Geometry check sheet. Reference: the model listing, model coordinates, mm. Face numbers are marked on the shaded views. A direction names the side the tool comes from. Round coordinates to 2 decimals unless told otherwise and drop trailing zeros. Loops run counter-clockwise (first coordinate to the right, second up) from the corner with the lowest first, then second, coordinate; pieces in that order, holes last. Notation, with made-up numbers: (86, 43.25) -> (99, 43.25) arc R15 ccw to (99, 61.25) -> close; hole circle Ø3 at (8.5, 18). An arc over 180 degrees is marked (long way). Use a Markdown table: item, result. Add a question column.
Q1. Sectioned sample at A-A, the plane y = 12.7. Enter the section's corners in (x, z) (3 decimals), then the cut area to 3 significant figures.
Q2. Sectioned sample at B-B, the plane x = 6.35. Enter the section's corners in (y, z) (3 decimals), then the cut area to 3 significant figures.
Q3. Set-up check for the marked faces 1, 2 and 3: record each of +Z, -Z, +X, -X, +Y, -Y from which the full face is reachable in a straight line by a thin tool's end or side.
Q4. Gauge pin test, flat ends, axial feed: P1, Ø3, axis at x = 6.35, z = -88.9, coming from the -Y side; P2, Ø12.5, axis at x = 16.5, y = 43, coming from the -Z side; P3, Ø8, axis at x = 12.5, z = -26, coming from the -Y side; P4, Ø10, axis at x = 4, z = -52, coming from the -Y side (3 decimals). Record the tip position at first contact, or that the pin passes through.
Q5. Sectioned sample at C-C, the plane z = -88.9. Enter the section's corners in (x, y) (3 decimals), then the cut area to 3 significant figures.
Q6. Material ranges on L1, parallel to X at y = 12.7, z = -1.8; L2, parallel to Y at x = 6.35, z = -2.5; L3, parallel to Z at x = 6.35, y = 100.7, recorded low to high.
Q7. Sectioned sample at D-D, the plane y = 93. Enter the section's corners in (x, z) (3 decimals), then the cut area to 3 significant figures.
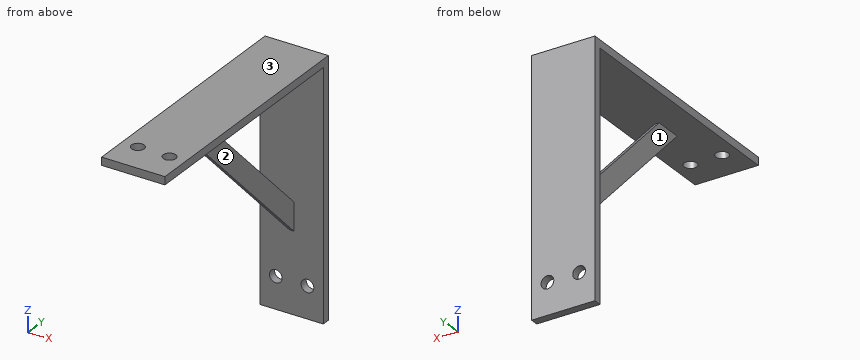
Autodesk Inventor part; units mm, degrees
ref_plane "Work Plane1" through (12.7, 0, 0) normal (1, 0, 0) x (0, 0, -1)
ref_plane "YZ Plane" through (0, 0, 0) normal (1, 0, 0) x (0, 1, 0)
ref_plane "XZ Plane" through (0, 0, 0) normal (0, 1, 0) x (-1, 0, 0)
sketch "Sketch1" plane through (0, 0, 0) normal (1, 0, 0) x (0, 1, 0)
  line L0 (0, 0) -> (101.6, 0)
  line L1 (101.6, 0) -> (101.6, -101.6)
  line L2 (98.425, -101.6) -> (98.425, -3.175)
  line L3 (98.425, -3.175) -> (0, -3.175)
  line L4 (101.6, -101.6) -> (98.425, -101.6)
  line L5 (0, 0) -> (0, -3.175)
  dimension "d0" = 101.6
  dimension "d1" = 101.6
  dimension "d2" = 3.175
extrude "Extrusion1" add sketch "Sketch1" along normal blind 25.4
ref_plane "Work Plane1" through (12.7, 0, 0) normal (1, 0, 0) x (0, 0, -1)
sketch "Sketch2" plane through (12.7, 0, 0) normal (1, 0, 0) x (0, 0, -1)
  line L0 (2.312, 31.3076) -> (70.5907, 99.5863)
  line L1 (2.312, 31.3076) -> (98.8727, 31.3076) construction
  line L2 (59.3736, 99.5863) -> (2.312, 42.5247)
  line L3 (70.5907, 99.5863) -> (59.3736, 99.5863)
  line L4 (2.312, 31.3076) -> (2.312, 42.5247)
  point P0 (0, 0)
  dimension "d6" = 45
  dimension "d7" = 7.9317
extrude "Extrusion2" add sketch "Sketch2" along normal mid plane 1.778
sketch "Sketch4" plane through (0, 98.425, -101.6) normal (0, -1, 0) x (1, 0, 0)
  line L0 (0, 0) -> (0, 98.425)
  line L1 (0, 0) -> (25.4, 0)
  circle A0 centre (6.35, 12.7) radius 2.2746
  circle A1 centre (19.05, 12.7) radius 2.2746
  point P0 (0, 101.6)
  dimension "d10" = 12.7
  dimension "d11" = 6.35
  dimension "d14" = 12.7
hole "Hole1" at (19.05, 98.425, -88.9) at (6.35, 98.425, -88.9) direction (0, 1, 0) diameter 5.1054 depth 25.4 tip angle 118
sketch "Sketch5" plane through (0, 0, -3.175) normal (0, 0, -1) x (-1, 0, 0)
  line L0 (-25.4, 0) -> (-25.4, 98.425)
  line L1 (0, 0) -> (-25.4, 0)
  circle A0 centre (-19.05, 12.7) radius 2.2861
  circle A1 centre (-6.35, 12.7) radius 2.2861
  dimension "d26" = 12.7
  dimension "d27" = 6.35
  dimension "d30" = 12.7
hole "Hole2" at (19.05, 12.7, -3.175) at (6.35, 12.7, -3.175) direction (0, 0, 1) diameter 5.1054 depth 25.4 tip angle 118
equation "\"d11\" = 0.25 * d3"
equation "\"d14\" = 0.5 * d3"
equation "\"d27\" = 0.25 * d3"
equation "\"d30\" = 0.5 * d3"
equation "\"d5\" = -0.5 * d3"
properties part number "angleBracket"
Values:
| question | item | result |
|---|---|---|
| 1 | outline | (0, -3.175) -> (3.797, -3.175) -> (3.797, 0) -> (0, 0) -> close; (8.903, -3.175) -> (16.497, -3.175) -> (16.497, 0) -> (8.903, 0) -> close; (21.603, -3.175) -> (25.4, -3.175) -> (25.4, 0) -> (21.603, 0) -> close |
| 1 | area | 48.2 mm^2 |
| 2 | outline | (0, -3.175) -> (10.147, -3.175) -> (10.147, 0) -> (0, 0) -> close; (15.253, -3.175) -> (98.425, -3.175) -> (98.425, -86.347) -> (101.6, -86.347) -> (101.6, 0) -> (15.253, 0) -> close; (98.425, -101.6) -> (101.6, -101.6) -> (101.6, -91.453) -> (98.425, -91.453) -> close |
| 2 | area | 603 mm^2 |
| 3 | face 1 | -Z, -X, -Y |
| 3 | face 2 | -Z, +X, -Y |
| 3 | face 3 | +Z, +X, -X, +Y, -Y |
| 4 | P1 | through |
| 4 | P2 | z = -19.54 |
| 4 | P3 | y = 51 |
| 4 | P4 | y = 98.425 |
| 5 | outline | (0, 98.425) -> (3.797, 98.425) -> (3.797, 101.6) -> (0, 101.6) -> close; (8.903, 98.425) -> (16.497, 98.425) -> (16.497, 101.6) -> (8.903, 101.6) -> close; (21.603, 98.425) -> (25.4, 98.425) -> (25.4, 101.6) -> (21.603, 101.6) -> close |
| 5 | area | 48.2 mm^2 |
| 6 | L1 | 0 to 3.8, 8.9 to 16.5, 21.6 to 25.4 |
| 6 | L2 | 0 to 10.15, 15.25 to 101.6 |
| 6 | L3 | -101.6 to -91.45, -86.35 to 0 |
| 7 | outline | (0, -3.175) -> (25.4, -3.175) -> (25.4, 0) -> (0, 0) -> close; (11.811, -64.004) -> (13.589, -64.004) -> (13.589, -52.787) -> (11.811, -52.787) -> close |
| 7 | area | 101 mm^2 |
